```python
from build123d import *

# Parameters (mm, degrees)
EXTRUDE_1_DEPTH     = 4
SKETCH_2_R          = 8
EXTRUDE_2_DEPTH     = 4
SKETCH_12_W         = 4
SKETCH_12_H         = 2
SKETCH_13_R         = 2
SKETCH_14_R         = 2
CUT_EXTRUDE_1_DEPTH = 1
SKETCH_15_R         = 2
CUT_EXTRUDE_2_DEPTH = 13


with BuildPart() as part:
    # 草图1 → 凸台-拉伸1 (new body)
    with BuildSketch(Plane.XY):
        with BuildLine():
            ThreePointArc((-12.158788541, 3.305126504), (0, -12.6), (12.158788541, 3.305126504))
            Line((12.158788541, 3.305126504), (5.366883622, 19.743511481))
            ThreePointArc((5.366883622, 19.743511481), (-0.204686635, 23.072677305), (-5.535757021, 19.370592925))
            Line((-5.535757021, 19.370592925), (-12.158788541, 3.305126504))
        make_face()
    extrude_1 = extrude(amount=EXTRUDE_1_DEPTH)

    # 草图2 → 凸台-拉伸2 (add)
    with BuildSketch(Plane.XY.offset(4)):
        Circle(SKETCH_2_R)
    extrude(amount=EXTRUDE_2_DEPTH)

    # 镜向1: 凸台-拉伸1 across plane
    add(extrude_1.mirror(Plane.XY.offset(6)))

    # 草图12 → 旋转3 (revolve)
    with BuildSketch(Plane(origin=(0, 0, 0), x_dir=(0, 0, -1), z_dir=(1, 0, 0))):
        with Locations((-6, 9)):
            Rectangle(SKETCH_12_W, SKETCH_12_H)
    revolve(axis=Axis((0, 0, -2.657619659), (0, 0, 1)))

    # 草图13 → 切除-旋转1 (revolve, cut)
    with BuildSketch(Plane(origin=(0, 0, 0), x_dir=(0, 0, -1), z_dir=(1, 0, 0))):
        with Locations((-6, 10)):
            Circle(SKETCH_13_R)
    revolve(axis=Axis((0, 0, -2.657619659), (0, 0, 1)), mode=Mode.SUBTRACT)

    # 草图14 → 切除-拉伸1 (cut)
    with BuildSketch(Plane(origin=(0, 0, 0), x_dir=(-1, 0, 0), z_dir=(0, 0, -1))):
        Circle(SKETCH_14_R)
    extrude(amount=-CUT_EXTRUDE_1_DEPTH, mode=Mode.SUBTRACT)

    # 草图15 → 切除-拉伸2 (cut, through all)
    with BuildSketch(Plane.XY.offset(12)):
        Circle(SKETCH_15_R)
    extrude(amount=-CUT_EXTRUDE_2_DEPTH, mode=Mode.SUBTRACT)


solid = part.part
```
Input: part model. Units: mm. Frame: model coordinates. Round coordinates to 2 decimals unless told otherwise and drop trailing zeros. Loops run counter-clockwise (first coordinate to the right, second up) from the corner with the lowest first, then second, coordinate; pieces in that order, holes last. Notation, with made-up numbers: M 52,-2 L 59,-2 A20 cw 59,21 Z; hole C -14,50 d6. An arc over 180 degrees is marked long. Answer in a Markdown table with one row per item. Add a question column.
1. Section C-C (z = 2.5). Output: boundary loops of the cut face in (x, y).
2. Mould query, pull axis Z, two halves, no side actions, for faces 1 (the face through (-0.109, 23.075, 1.972)), 2 (the face through (0, 5, 0)), 3 (the face through (5, 9, 8)), 4 (the face through (5, 9, 4)). Classes: released by +Z, released by -Z, zero draft, split by the parting line, or undercut.
3. Section B-B (x = 0). Output: boundary loops of the cut face in (y, z), and give its area (3 significant figures).
4. Ray query, probe 1 along Z at (x, y) = (-5.75, 13.5); probe 2 along Y at (x, z) = (0, 8.25); probe 3 along X at (y, z) = (1, 5.25). Return the intervals inside material, ascending.
5. Section D-D (y = 12.5). Output: boundary loops of the cut face in (x, z).
6. Section A-A (y = 0). Output: boundary loops of the cut face in (x, z).
7. Contact query for flat-ended pins moving along their axis: pin 1 (1 mm diameter, centred on y = 10.5, z = 3, fed in from -X); pin 2 (1 mm diameter, centred on x = -7, z = 1.5, fed in from -Y); pin 3 (5 mm diameter, centred on x = -5, z = 3.5, fed in from +Y); pin 4 (10 mm diameter, centred on x = 1, y = 4, fed in from -Z). Output: stop coordinate, or through.
Values follow:
| question | item | result |
|---|---|---|
| 1 | outline | M -12.16,3.31 A12.6 ccw long 12.16,3.31 L 5.37,19.74 A5.99 ccw -5.54,19.37 Z; hole C 0,0 d4 |
| 2 | face 1 | zero draft |
| 2 | face 2 | released by -Z |
| 2 | face 3 | undercut |
| 2 | face 4 | undercut |
| 3 | outline | M -12.6,0 L -2,0 L -2,12 L -12.6,12 L -12.6,8 L -10,8 A2 cw -10,4 L -12.6,4 Z; M 2,0 L 23.08,0 L 23.08,4 L 10,4 A2 cw 10,8 L 23.08,8 L 23.08,12 L 2,12 Z |
| 3 | area | 305 mm^2 |
| 4 | probe 1 | 0 to 4, 8 to 12 |
| 4 | probe 2 | -12.6 to -2, 2 to 23.08 |
| 4 | probe 3 | -8.08 to -1.73, 1.73 to 8.08 |
| 5 | outline | M -8.37,0 L 8.36,0 L 8.36,4 L -8.37,4 Z; M -8.37,8 L 8.36,8 L 8.36,12 L -8.37,12 Z |
| 6 | outline | M -12.6,0 L -2,0 L -2,12 L -12.6,12 L -12.6,8 L -10,8 A2 cw -10,4 L -12.6,4 Z; M 2,0 L 12.6,0 L 12.6,4 L 10,4 A2 cw 10,8 L 12.6,8 L 12.6,12 L 2,12 Z |
| 7 | pin 1 | x = -9.4 |
| 7 | pin 2 | y = -10.79 |
| 7 | pin 3 | y = 22.53 |
| 7 | pin 4 | z = 0 |
